The model under review builds one solid part; all positions refer to its coordinate system, in mm. A direction names the side the tool comes from. Round coordinates to 2 decimals unless told otherwise and drop trailing zeros. Write each loop counter-clockwise with the first axis right and the second up, starting at its lowest first coordinate (ties: lowest second). Pieces come first, ordered by that corner, then holes. Notation, with made-up numbers: (18, 48.25) - (48, 48.25) arc R24 cw to (48, 80.25) - close; hole circle Ø6 at (24, 66.5). An arc over 180 degrees is marked (long way). Use one line per item in the form item = value.
from build123d import *

# Parameters (mm, degrees)
CROQUIS1_W              = 5
CROQUIS1_H              = 30
SALIENTE_EXTRUIR1_DEPTH = 15
CROQUIS2_R              = 3.5
CORTAR_EXTRUIR1_DEPTH   = 15
CROQUIS3_W              = 5
CROQUIS3_H              = 17
SALIENTE_EXTRUIR2_DEPTH = 80
CROQUIS5_R              = 2
CORTAR_EXTRUIR3_DEPTH   = 75
CORTAR_EXTRUIR4_DEPTH   = 30


with BuildPart() as part:
    # Croquis1 → Saliente-Extruir1 (new body)
    with BuildSketch(Plane.XY):
        Rectangle(CROQUIS1_W, CROQUIS1_H)
    extrude(amount=SALIENTE_EXTRUIR1_DEPTH)

    # Croquis2 → Cortar-Extruir1 (cut)
    with BuildSketch(Plane(origin=(2.5, 0, 0), x_dir=(0, 0, -1), z_dir=(1, 0, 0))):
        with Locations((-7.5, 9.795077014)):
            Circle(CROQUIS2_R)
        with Locations((-7.5, -10.204922986)):
            Circle(CROQUIS2_R)
    extrude(amount=-CORTAR_EXTRUIR1_DEPTH, mode=Mode.SUBTRACT)

    # Croquis3 → Saliente-Extruir2 (add)
    with BuildSketch(Plane(origin=(0, 0, 0), x_dir=(-1, 0, 0), z_dir=(0, 0, -1))):
        with Locations((0, -6.5)):
            Rectangle(CROQUIS3_W, CROQUIS3_H)
    extrude(amount=SALIENTE_EXTRUIR2_DEPTH)

    # Croquis5 → Cortar-Extruir3 (cut)
    with BuildSketch(Plane(origin=(2.5, 0, 0), x_dir=(0, 0, -1), z_dir=(1, 0, 0))):
        with Locations((65, -6.5)):
            Circle(CROQUIS5_R)
        with Locations((55, -6.5)):
            Circle(CROQUIS5_R)
    extrude(amount=-CORTAR_EXTRUIR3_DEPTH, mode=Mode.SUBTRACT)

    # Croquis6 → Cortar-Extruir4 (cut)
    with BuildSketch(Plane(origin=(0, 2, 0), x_dir=(1, 0, 0), z_dir=(0, 1, 0))):
        Polygon((-2.5, 70), (2.5, 75), (2.5, 80), (-2.5, 80), align=None)
    extrude(amount=-CORTAR_EXTRUIR4_DEPTH, mode=Mode.SUBTRACT)


solid = part.part
(1) Add section D-D on y = -0.5. Write out the cut boundary in (x, z), then the cut area to 4 significant figures.
Geometry results:
outline = (-2.5, -70) - (2.5, -75) - (2.5, 15) - (-2.5, 15) - close
area = 437.5 mm2
(2) Add section C-C on x = 0.25. Write out the cut boundary in (y, z).
Geometry results:
outline = (-15, -72.75) - (2, -72.75) - (2, 0) - (15, 0) - (15, 15) - (-15, 15) - close; hole circle Ø7 at (-10.2, 7.5); hole circle Ø4 at (-6.5, -65); hole circle Ø4 at (-6.5, -55); hole circle Ø7 at (9.8, 7.5)
(3) Insertion check: P1, Ø5, axis at y = -6.5, z = -55, coming from the -X side; P2, Ø2.5, axis at x = 1, y = 6, coming from the -Z side. Each pin has a flat end and moves straight along its axis. Give the tip position at first contact, or say it passes through.
Geometry results:
P1 = -2.5
P2 = 0
(4) To check wall thickness, follow L1, parallel to Y at x = 1.25, z = -65; L2, parallel to Y at x = -1.05, z = 5; L3, parallel to Z at x = 1.1, y = 4.25. State the ranges of each line that lie inside material, in increasing order.
Geometry results:
L1 = -15 to -8.5, -4.5 to 2
L2 = -15 to -12.65, -7.76 to 7.35, 12.24 to 15
L3 = 0 to 15
(5) Add section A-A on z = -55. Write out the cut boundary in (x, y).
Geometry results:
outline = (-2.5, -15) - (2.5, -15) - (2.5, -8.5) - (-2.5, -8.5) - close; (-2.5, -4.5) - (2.5, -4.5) - (2.5, 2) - (-2.5, 2) - close
(6) Machinability: for faces 1 (the flat face through (0, 9, 0)), 2 (the flat face through (2.5, -4, -29)), which of the approach directions +Z, -Z, +X, -X, +Y, -Y give a long, thin tool a straight path to every point of the face, cutting with its end or side? Answer none if there is none.
Geometry results:
face_1 = -Z, +X, -X, +Y
face_2 = +Z, -Z, +X, +Y, -Y
(7) Add section B-B on y = -11. Write out the cut boundary in (x, z), then the cut area to 3 significant figures.
Geometry results:
outline = (-2.5, -70) - (2.5, -75) - (2.5, 4.09) - (-2.5, 4.09) - close; (-2.5, 10.91) - (2.5, 10.91) - (2.5, 15) - (-2.5, 15) - close
area = 403 mm2
(8) The part is to be moulded in two halves that separate along Y. For faces 3 (the flat face through (0, -15, -29)), 4 (the cylindrical face through (0, 9.9, 11)), 5 (the flat face through (0, 2, -37)), say which applies: +Y half, -Y half, draft (parallel to the pull), parting line (faces both ways), or undercut.
Geometry results:
face_3 = -Y half
face_4 = undercut
face_5 = +Y half
